```python
from build123d import *

# Parameters (mm, degrees)
SKETCH_W         = 45
SKETCH_H         = 45
SKETCH_R         = 18.5
PAD_DEPTH        = 6
SKETCH001_R      = 18.5
SKETCH001_R_2    = 9
PAD001_DEPTH     = 0.6
POCKET_DEPTH     = 5.65
HOLE_D           = 2.3
HOLE_DEPTH       = 9.4
HOLE_CSINK_D     = 3.5
HOLE_CSINK_ANGLE = 90
CHAMFER_SIZE     = 2
CHAMFER001_SIZE  = 1
SKETCH004_W      = 12.5
SKETCH004_H      = 25
POCKET002_DEPTH  = 6.3
POCKET006_DEPTH  = 7.5
CHAMFER003_SIZE  = 0.6


with BuildPart() as part:
    # Sketch → Pad (new body)
    with BuildSketch(Plane.XY):
        Rectangle(SKETCH_W, SKETCH_H)
        Circle(SKETCH_R, mode=Mode.SUBTRACT)
    extrude(amount=PAD_DEPTH)

    # Sketch001 → Pad001 (join)
    with BuildSketch(Plane.XY):
        Circle(SKETCH001_R)
        Circle(SKETCH001_R_2, mode=Mode.SUBTRACT)
    extrude(amount=PAD001_DEPTH)

    # Sketch002 → Pocket (cut)
    with BuildSketch(Plane.XY.offset(10)):
        with BuildLine():
            ThreePointArc((19.851008, 4), (0, 20.25), (-19.851008, 4))
            Line((-20.831304, 4.197531), (-19.851008, 4))
            ThreePointArc((-20.831304, 4.197531), (-21.25, 0), (-20.831304, -4.197531))
            Line((-20.831304, -4.197531), (-19.851008, -4))
            ThreePointArc((-19.851008, -4), (-14.318912, -14.318912), (-4, -19.851008))
            Line((-4.197531, -20.831304), (-4, -19.851008))
            ThreePointArc((-4.197531, -20.831304), (0, -21.25), (4.197531, -20.831304))
            Line((4.197531, -20.831304), (4, -19.851008))
            ThreePointArc((4, -19.851008), (14.318912, -14.318912), (19.851008, -4))
            Line((19.851008, -4), (20.831304, -4.197531))
            ThreePointArc((20.831304, -4.197531), (21.25, 0), (20.831304, 4.197531))
            Line((19.851008, 4), (20.831304, 4.197531))
        make_face()
    extrude(amount=-POCKET_DEPTH, mode=Mode.SUBTRACT)

    # Hole
    with Locations(Plane.XY.offset(10)):
        with Locations((-17, 17), (-17, -17), (17, -17), (17, 17)):
            CounterSinkHole(HOLE_D / 2, HOLE_CSINK_D / 2, depth=HOLE_DEPTH, counter_sink_angle=HOLE_CSINK_ANGLE)

    # Chamfer
    chamfer_edges = [part.edges().sort_by_distance(p)[0] for p in [
        (22.5, -22.5, 3),
        (-22.5, -22.5, 3),
        (22.5, 22.5, 3),
        (-22.5, 22.5, 3),
    ]]
    chamfer(chamfer_edges, length=CHAMFER_SIZE)

    # Chamfer001
    chamfer001_edges = [part.edges().sort_by_distance(p)[0] for p in [
        (0, 22.5, 0),
        (-22.5, 0, 0),
        (-21.5, 21.5, 0),
        (22.5, 0, 0),
        (-21.5, -21.5, 0),
        (21.5, 21.5, 0),
        (0, -22.5, 0),
        (21.5, -21.5, 0),
    ]]
    chamfer(chamfer001_edges, length=CHAMFER001_SIZE)

    # Sketch004 → Pocket002 (cut)
    with BuildSketch(Plane.XY.offset(10)):
        with Locations((0, 12.5)):
            Rectangle(SKETCH004_W, SKETCH004_H)
    extrude(amount=-POCKET002_DEPTH, mode=Mode.SUBTRACT)

    # Sketch006 → Pocket006 (cut)
    with BuildSketch(Plane.XY.offset(10)):
        with BuildLine():
            Line((-13.175878, 15.377215), (-11.711892, 13.668635))
            ThreePointArc((-7.5, 16.363068), (-9.699958, 15.16281), (-11.711892, 13.668635))
            Line((-8.4375, 18.408452), (-7.5, 16.363068))
            ThreePointArc((-8.4375, 18.408452), (-10.912453, 17.058161), (-13.175878, 15.377215))
        make_face()
    extrude(amount=-POCKET006_DEPTH, mode=Mode.SUBTRACT)

    # Chamfer003
    chamfer003_edges = [part.edges().sort_by_distance(p)[0] for p in [
        (15.85, -17, 6),
        (-18.15, -17, 6),
        (-18.15, 17, 6),
        (15.85, 17, 6),
    ]]
    chamfer(chamfer003_edges, length=CHAMFER003_SIZE)


solid = part.part
```
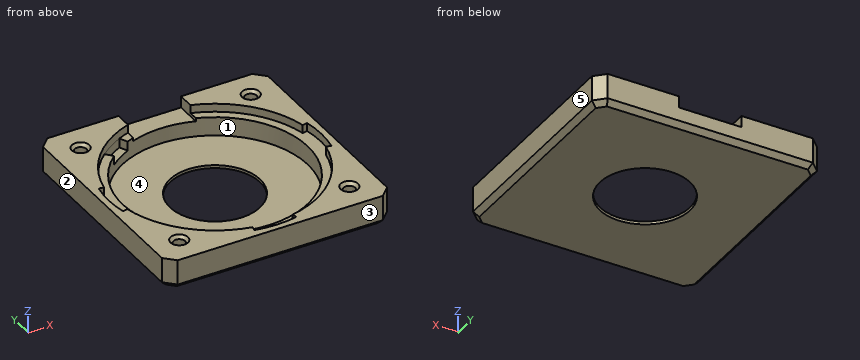
The model under review builds one solid part; all positions refer to its coordinate system, in mm. Face numbers are marked on the shaded views. A direction names the side the tool comes from. Round coordinates to 2 decimals unless told otherwise and drop trailing zeros. Order: outer loops, then holes, each group sorted by start corner. A loop starts at its lowest first (then second) coordinate and runs counter-clockwise, first axis right, second up.
Item 1: Machinability: for the marked faces 4 and 5, which of the approach directions +Z, -Z, +X, -X, +Y, -Y give a long, thin tool a straight path to every point of the face, cutting with its end or side? Answer none if there is none.
Working result:
face 4: +Z
face 5: +Z, -Z, +X, +Y, -Y
Item 2: For pin 1 (18.5 mm diameter, centred on x = 5.5, y = 4, fed in from +Z); pin 2 (2.5 mm diameter, centred on x = 2, y = 20, fed in from +Z); pin 3 (1.8 mm diameter, centred on x = 17.5, y = 17, fed in from +Z), all flat-tipped, find the tip position at first contact; note any pin that passes through.
Working result:
pin 1: stops at z = 0.6
pin 2: stops at z = 3.7
pin 3: stops at z = 5.65
Item 3: Add section A-A, the plane y = 0. State the section outline as (x, z) points.
Working result:
outline: (-22.5, 1) - (-21.5, 0) - (-9, 0) - (-9, 0.6) - (-18.5, 0.6) - (-18.5, 4.35) - (-21.25, 4.35) - (-21.25, 6) - (-22.5, 6) - close; (9, 0) - (21.5, 0) - (22.5, 1) - (22.5, 6) - (21.25, 6) - (21.25, 4.35) - (18.5, 4.35) - (18.5, 0.6) - (9, 0.6) - close
Item 4: Add section B-B, the plane z = 1.9. State the section outline as (x, y) points.
Working result:
outline: (-22.5, -20.5) - (-20.5, -22.5) - (20.5, -22.5) - (22.5, -20.5) - (22.5, 20.5) - (20.5, 22.5) - (-20.5, 22.5) - (-22.5, 20.5) - close; hole circle Ø37 at (0, 0); hole circle Ø2.3 at (-17, -17); hole circle Ø2.3 at (-17, 17); hole circle Ø2.3 at (17, -17); hole circle Ø2.3 at (17, 17)
Item 5: Draft analysis for pull direction X (two halves, no side actions). For the marked faces 1, 2 and 3, state which applies: released by +X, released by -X, zero draft, split by the parting line, or undercut.
Working result:
face 1: undercut
face 2: released by -X
face 3: zero draft
Item 6: Add section C-C, the plane x = 0. State the section outline as (y, z) points, and give its area (3 significant figures).
Working result:
outline: (-22.5, 1) - (-21.5, 0) - (-9, 0) - (-9, 0.6) - (-18.5, 0.6) - (-18.5, 4.35) - (-21.25, 4.35) - (-21.25, 6) - (-22.5, 6) - close; (9, 0) - (21.5, 0) - (22.5, 1) - (22.5, 3.7) - (18.5, 3.7) - (18.5, 0.6) - (9, 0.6) - close
area: 44.7 mm2
Item 7: Add section D-D, the plane x = 17. State the section outline as (y, z) points.
Working result:
outline: (-22.5, 1) - (-21.5, 0) - (21.5, 0) - (22.5, 1) - (22.5, 6) - (18.75, 6) - (18.15, 5.4) - (18.15, 0.6) - (15.85, 0.6) - (15.85, 5.4) - (15.25, 6) - (11, 6) - (11, 4.35) - (7.3, 4.35) - (7.3, 0.6) - (-7.3, 0.6) - (-7.3, 4.35) - (-11, 4.35) - (-11, 6) - (-15.25, 6) - (-15.85, 5.4) - (-15.85, 0.6) - (-18.15, 0.6) - (-18.15, 5.4) - (-18.75, 6) - (-22.5, 6) - close
Item 8: To check wall thickness, follow probe 1 along Y at (x, z) = (0, 1.4); probe 2 along Y at (x, z) = (-17, 3.4); probe 3 along Z at (x, y) = (8, -13). State the ranges of each line that lie inside material, in increasing order.
Working result:
probe 1: y = -22.5 to -18.5, 18.5 to 22.5
probe 2: y = -22.5 to -18.15, -15.85 to -7.3, 7.3 to 15.85, 18.15 to 22.5
probe 3: z = 0 to 0.6
